Here's how the part is built. I have some questions about the finished solid (model axes, mm). A direction names the side the tool comes from. Give positions to 0.01 mm unless a question says otherwise; leave off trailing zeros. Write each loop counter-clockwise with the first axis right and the second up, starting at its lowest first coordinate (ties: lowest second). Pieces come first, ordered by that corner, then holes. Notation, with made-up numbers: (-29.5, -4) - (23.5, -4) arc R27 cw to (23.5, 27) - close; hole circle Ø7 at (5.25, 59.5). An arc over 180 degrees is marked (long way). Write each question's results on one line, items separated by ' | '. Start each with the question number.
Item 1: We'd pull the mould along Z, two halves only. Please class faces 1 (the flat face through (21.15, 4, -11)), 2 (the flat face through (-17, 2, 21.15)), 3 (the cylindrical face through (-17, 2.54, -15.57)): +Z half, -Z half, draft (parallel to the pull), parting line (faces both ways), or undercut.
Item 2: Suppose I cut it at A-A on x = 15.5. List the corners of the cut face in (y, z) for me.
Item 3: Suppose I cut it at D-D on z = -15.5. List the corners of the cut face in (x, y) for me, then the cut area to 3 significant figures.
Item 4: Suppose I cut it at C-C on x = -42.3. List the corners of the cut face in (y, z) for me.
Item 5: Suppose I cut it at B-B on z = 0. List the corners of the cut face in (x, y) for me, then the cut area to 3 significant figures.
Item 6: Will these pins go through, and if not, where does the flat tip stop? P1, Ø1.5, axis at y = 25, z = -25, coming from the -X side; P2, Ø3, axis at x = -32.5, z = 16.5, coming from the +Y side; P3, Ø1.5, axis at x = -45.5, y = 3, coming from the -Z side.
Item 7: Which directions (+Z, -Z, +X, -X, +Y, -Y) give clear straight access to the entire face, cutting with the end or side of a thin tool? Please do faces 4 (the flat face through (-45, 2, -21.15)), 5 (the flat face through (-16, 5, 0)), 6 (the flat face through (-7, 22, -26.15)).
Item 8: Please list where these lines run through material, in increasing order: line 1 along X through (y, z) = (2.3, -15.5); line 2 along Z through (x, y) = (-42.3, 1.8); line 3 along X through (y, z) = (1, -15).
Autodesk Inventor part; units mm, degrees
ref_plane "Plano de trabajo1" through (0, -17, 0) normal (0, -1, 0) x (1, 0, 0)
ref_plane "YZ Plane" through (0, 0, 0) normal (1, 0, 0) x (0, 1, 0)
ref_plane "XZ Plane" through (0, 0, 0) normal (0, 1, 0) x (-1, 0, 0)
sketch "Boceto1" plane through (0, 0, 0) normal (0, 1, 0) x (-1, 0, 0)
  line L0 (21.15, 21.15) -> (-21.15, 21.15)
  line L1 (-21.15, 21.15) -> (-21.15, -21.15)
  line L2 (-21.15, -21.15) -> (21.15, -21.15)
  line L3 (21.15, -21.15) -> (21.15, 21.15)
  line L4 (0, 0) -> (3.2885, 0)
  line L5 (0, 0) -> (0, -4.7563)
  circle A0 centre (0, 0) radius 11.5
  line L6 (21.15, -21.15) -> (55, -21.15)
  line L7 (55, -21.15) -> (55, 21.15)
  line L8 (55, 21.15) -> (21.15, 21.15)
  line L9 (21.15, 21.15) -> (21.15, -21.15)
  dimension "d0" = 42.3
  dimension "d1" = 42.3
  dimension "d26" = 23
  dimension "d35" = 55
extrude "Extrusión1" add sketch "Boceto1" along normal blind 5
sketch "Boceto2" plane through (0, 5, 0) normal (0, 1, 0) x (1, 0, 0)
  circle A0 centre (-15.5, 15.5) radius 1.5
  point P0 (0, 0)
  dimension "d4" = 3
  dimension "d5" = 15.5
  dimension "d6" = 15.5
extrude "Extrusión2" cut sketch "Boceto2" against normal through all
pattern_circular "Patrón circular1" count 4 over 360 about axis through (0, -10, 0) along (0, 1, 0) of "Extrusión2"
sketch "Boceto7" plane through (0, 0, 0) normal (0, -1, 0) x (1, 0, 0)
  circle A0 centre (-42.3, 0) radius 2
  point P0 (0, 0)
  dimension "d31" = 4
  dimension "d32" = 42.3
extrude "Extrusión7" cut sketch "Boceto7" against normal through all
sketch "Boceto8" plane through (21.15, 0, -21.15) normal (0, 0, -1) x (-1, 0, 0)
  line L0 (0, 0) -> (0, 5)
  line L1 (0, 0) -> (56.15, 0)
  line L2 (56.15, 0) -> (56.15, 44)
  line L3 (56.15, 44) -> (0, 44)
  line L4 (0, 44) -> (0, 0)
  line L5 (0, 5) -> (76.15, 5)
  point P0 (21.15, 0)
  dimension "d36" = 39
extrude "Extrusión8" add sketch "Boceto8" along normal blind 5
ref_plane "Plano de trabajo1" through (0, -17, 0) normal (0, -1, 0) x (1, 0, 0)
equation "\"d0\" = d1"
properties part number "Base Motor X1"
Checked values:
1) face 1: draft | face 2: +Z half | face 3: undercut
2) outline: (0, -26.15) - (44, -26.15) - (44, -21.15) - (5, -21.15) - (5, -17) - (0, -17) - close; (0, -14) - (5, -14) - (5, 14) - (0, 14) - close; (0, 17) - (5, 17) - (5, 21.15) - (0, 21.15) - close
3) outline: (-55, 0) - (-17, 0) - (-17, 5) - (-55, 5) - close; (-14, 0) - (14, 0) - (14, 5) - (-14, 5) - close; (17, 0) - (21.15, 0) - (21.15, 5) - (17, 5) - close | area: 351 mm^2
4) outline: (0, -21.15) - (5, -21.15) - (5, -2) - (0, -2) - close; (0, 2) - (5, 2) - (5, 21.15) - (0, 21.15) - close
5) outline: (-55, 0) - (-44.3, 0) - (-44.3, 5) - (-55, 5) - close; (-40.3, 0) - (-11.5, 0) - (-11.5, 5) - (-40.3, 5) - close; (11.5, 0) - (21.15, 0) - (21.15, 5) - (11.5, 5) - close | area: 246 mm^2
6) P1: stops at x = -35 | P2: stops at y = 5 | P3: stops at z = -21.15
7) face 4: -Z, -X, +Y, -Y | face 5: +Z, +X, -X, +Y | face 6: -Z, +X, -X, +Y, -Y
8) line 1: x = -55 to -17, -14 to 14, 17 to 21.15 | line 2: z = -21.15 to -2, 2 to 21.15 | line 3: x = -55 to -16.91, -14.09 to 14.09, 16.91 to 21.15
